from build123d import *

# Parameters (mm, degrees)
BRANCH_HUB_START       = -13
SKETCH1_R              = 6
BRANCH_HUB_DEPTH       = 13
RUN_BACK_PORT_START    = -20
SKETCH2_R              = 6
RUN_BACK_PORT_DEPTH    = 12
RUN_BACK_SOCKET_START  = -20
SKETCH3_R              = 3.2
RUN_BACK_SOCKET_DEPTH  = 10
RUN_FRONT_PORT_START   = 8
SKETCH4_R              = 6
RUN_FRONT_PORT_DEPTH   = 12
RUN_FRONT_SOCKET_START = 20
SKETCH5_R              = 3.2
RUN_FRONT_SOCKET_DEPTH = 10
RUN_HUB_START          = -8
SKETCH6_R              = 6
RUN_HUB_DEPTH          = 16
BRANCH_PORT_START      = -25
SKETCH7_R              = 6
BRANCH_PORT_DEPTH      = 12
BRANCH_SOCKET_START    = -25
SKETCH8_R              = 3.2
BRANCH_SOCKET_DEPTH    = 10


with BuildPart() as part:
    # Sketch1 → Branch_Hub (new body)
    with BuildSketch(Plane(origin=(0, 0, 0), x_dir=(0, 0, -1), z_dir=(1, 0, 0)).offset(BRANCH_HUB_START)):
        Circle(SKETCH1_R)
    extrude(amount=BRANCH_HUB_DEPTH)



with BuildPart() as body_2:
    # Sketch2 → Run_Back_Port (new body)
    with BuildSketch(Plane.XY.offset(RUN_BACK_PORT_START)):
        Circle(SKETCH2_R)
    extrude(amount=RUN_BACK_PORT_DEPTH)

    # Sketch3 → Run_Back_Socket (cut)
    with BuildSketch(Plane.XY.offset(RUN_BACK_SOCKET_START)):
        Circle(SKETCH3_R)
    extrude(amount=RUN_BACK_SOCKET_DEPTH, mode=Mode.SUBTRACT)


with BuildPart() as body_3:
    # Sketch4 → Run_Front_Port (new body)
    with BuildSketch(Plane.XY.offset(RUN_FRONT_PORT_START)):
        Circle(SKETCH4_R)
    extrude(amount=RUN_FRONT_PORT_DEPTH)

    # Sketch5 → Run_Front_Socket (cut)
    with BuildSketch(Plane.XY.offset(RUN_FRONT_SOCKET_START)):
        Circle(SKETCH5_R)
    extrude(amount=-RUN_FRONT_SOCKET_DEPTH, mode=Mode.SUBTRACT)


with BuildPart() as part_1:
    add(part.part)

    add(body_2.part)  # Run_Hub merges body 2

    add(body_3.part)  # Run_Hub merges body 3
    # Sketch6 → Run_Hub (add)
    with BuildSketch(Plane.XY.offset(RUN_HUB_START)):
        Circle(SKETCH6_R)
    extrude(amount=RUN_HUB_DEPTH)

    # Sketch7 → Branch_Port (add)
    with BuildSketch(Plane(origin=(0, 0, 0), x_dir=(0, 0, -1), z_dir=(1, 0, 0)).offset(BRANCH_PORT_START)):
        with Locations(Location((0, 0, 0), (0, 0, 90))):
            Circle(SKETCH7_R)
    extrude(amount=BRANCH_PORT_DEPTH)

    # Sketch8 → Branch_Socket (cut)
    with BuildSketch(Plane(origin=(0, 0, 0), x_dir=(0, 0, -1), z_dir=(1, 0, 0)).offset(BRANCH_SOCKET_START)):
        Circle(SKETCH8_R)
    extrude(amount=BRANCH_SOCKET_DEPTH, mode=Mode.SUBTRACT)


solid = part_1.part
Here's how the part is built. I have some questions about the finished solid (model axes, mm). A direction names the side the tool comes from. Round coordinates to 2 decimals unless told otherwise and drop trailing zeros. Write each loop counter-clockwise with the first axis right and the second up, starting at its lowest first coordinate (ties: lowest second). Pieces come first, ordered by that corner, then holes. Notation, with made-up numbers: (39.25, -7) -> (80.25, -7) arc R23 cw to (80.25, 9) -> close; hole circle Ø11 at (2, 80.25). An arc over 180 degrees is marked (long way). One line per item, written item: value.
1) We'd pull the mould along Y, two halves only. Please class faces 4 (the face through (0, 0, 10)), 5 (the face through (3, -3, -20)), 6 (the face through (5.723, 1.802, -0.28)): released by +Y, released by -Y, zero draft, split by the parting line, or undercut.
Filled sheet:
face 4: undercut
face 5: zero draft
face 6: split by the parting line
2) Suppose I cut it at C-C on x = -9. List the corners of the cut face in (y, z) for me, plus the area to 3 significant figures.
Filled sheet:
outline: circle Ø12 at (0, 0)
area: 113 mm2
3) If I drill on line 1 (Y direction, x = 0, z = -18); line 2 (Y direction, x = -2, z = -16); line 3 (Z direction, x = 2, y = -0.75), over which ranges is the centre line in solid material (lowest first)? Write a range as [from, to].
Filled sheet:
line 1: y = [-6, -3.2], [3.2, 6]
line 2: y = [-5.66, -2.5], [2.5, 5.66]
line 3: z = [-10, 10]
4) Suppose I cut it at B-B on y = -4.75. List the corners of the cut face in (x, z) for me, plus the area to 3 significant figures.
Filled sheet:
outline: (-25, -3.67) -> (-3.67, -3.67) -> (-3.67, -20) -> (3.67, -20) -> (3.67, 20) -> (-3.67, 20) -> (-3.67, 3.67) -> (-25, 3.67) -> close
area: 450 mm2
5) For faces 1 (the face through (0, 0, -10)), 2 (the face through (-15, 0, 0)), 3 (the face through (-2.539, -1.947, 15.07)), which set-ups out of +Z, -Z, +X, -X, +Y, -Y let a thin tool reach every point of the face, with its end or its side?
Filled sheet:
face 1: -Z
face 2: -X
face 3: +Z
6) Suppose I cut it at A-A on z = 10.5. List the corners of the cut face in (x, y) for me, plus the area to 3 significant figures.
Filled sheet:
outline: circle Ø12 at (0, 0); hole circle Ø6.4 at (0, 0)
area: 80.9 mm2
7) I'm going to push flat-ended pins straight in: pin 1 Ø3 at (y, z) = (-1, -1) entering from -X; pin 2 Ø1.5 at (x, y) = (-12, 4.5) entering from +Z; pin 3 Ø4 at (y, z) = (-2.5, 11.5) entering from -X. Where does each tip first touch, or does it pass through?
Filled sheet:
pin 1: stops at x = -15
pin 2: stops at z = 4.68
pin 3: stops at x = -5.98
